```python
from build123d import *

# Parameters (mm, degrees)
F0_R     = 117.5
F1_DEPTH = 12.5
F3_DEPTH = 12.5
F4_COUNT = 4


with BuildPart() as f1:
    # F0 (on Front) → F1 (new body, symmetric)
    with BuildSketch(Plane.XZ):
        Circle(F0_R)
    extrude(amount=F1_DEPTH, both=True)

    # F2 (on Front) → F3 (cut, symmetric)
    with BuildSketch(Plane.XZ):
        with BuildLine():
            Line((7.3289173795, 97.9024141661), (11.9843448736, 116.8872340247))
            ThreePointArc((11.9843448736, 116.8872340247), (0, 117.5), (-11.9843448736, 116.8872340247))
            Line((-11.9843448736, 116.8872340247), (-7.3289173795, 97.9024141661))
            ThreePointArc((-7.3289173795, 97.9024141661), (-5.5587216743, 95.1591403196), (-2.4727905872, 94.0932258964))
            Line((-2.4727905872, 94.0932258964), (2.4727905872, 94.0932258964))
            ThreePointArc((2.4727905872, 94.0932258964), (5.5587216743, 95.1591403196), (7.3289173795, 97.9024141661))
        make_face()
    f3 = extrude(amount=F3_DEPTH, both=True, mode=Mode.SUBTRACT)

    # F4: F3 ×4 about axis
    f4_axis = Axis((0, 0, 0), (0, -1, 0))
    for i in range(1, F4_COUNT):
        add(f3.rotate(f4_axis, i * 360 / F4_COUNT), mode=Mode.SUBTRACT)


solid = f1.part
```
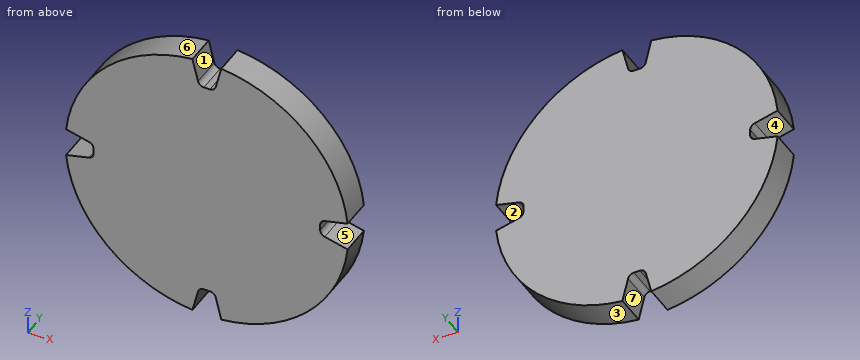
Can you work these out from the model? Positions are in its coordinate system, mm. Face numbers are marked on the shaded views. A direction names the side the tool comes from. Coordinates: 2 decimals unless noted, no trailing zeros. Loops run counter-clockwise (first coordinate to the right, second up) from the corner with the lowest first, then second, coordinate; pieces in that order, holes last.
1) For pin 1 (2.5 mm diameter, centred on y = -1, z = -0.5, fed in from -X); pin 2 (5 mm diameter, centred on x = 60.5, y = -9, fed in from +Z); pin 3 (2 mm diameter, centred on x = 74, y = 1.5, fed in from +Z), each with a flat end and sliding along its axis, tell me the tip position at first contact or that it passes through.
2) Thinking about a two-plate mould opening in X: for the marked faces 5, 6 and 7, which applies, pulls with the +X half, pulls with the -X half, needs draft (parallel to the pull), parting line crosses it, or undercut?
3) Imagine slicing it at C-C on z = 72. List the corners of the cut face in (x, y) for me, plus the area to 3 significant figures.
4) I need wall thicknesses on probe 1 along X at (y, z) = (-7.25, 1.5); probe 2 along Z at (x, y) = (107.5, 10.5); probe 3 along X at (y, z) = (-8.5, 106). Which ranges of each line are inside material? Lowest first, please.
5) Which directions (+Z, -Z, +X, -X, +Y, -Y) give clear straight access to the entire face, cutting with the end or side of a thin tool? Please do the marked faces 1, 2, 3 and 4.
6) Imagine slicing it at B-B on x = 39.5. List the corners of the cut face in (y, z) for me, plus the area to 3 significant figures.
7) Imagine slicing it at A-A on y = -9.25. List the corners of the cut face in (x, z) for me, plus the area to 3 significant figures.
Completed:
1. pin 1: stops at x = -94.09
1. pin 2: stops at z = 102.19
1. pin 3: stops at z = 92.07
2. face 5: pulls with the +X half
2. face 6: pulls with the -X half
2. face 7: undercut
3. outline: (-92.86, -12.5) - (92.86, -12.5) - (92.86, 12.5) - (-92.86, 12.5) - close
3. area: 4,640 mm2
4. probe 1: x = -94.09 to 94.09
4. probe 2: z = -47.43 to -9.68, 9.68 to 47.43
4. probe 3: x = -50.7 to -9.31, 9.31 to 50.7
5. face 1: +Z, +Y, -Y
5. face 2: +X, +Y, -Y
5. face 3: -Z, +X, +Y, -Y
5. face 4: -X, +Y, -Y
6. outline: (-12.5, -110.66) - (12.5, -110.66) - (12.5, 110.66) - (-12.5, 110.66) - close
6. area: 5,530 mm2
7. outline: (-116.89, -11.98) arc R117.5 ccw to (-11.98, -116.89) - (-7.33, -97.9) arc R5 cw to (-2.47, -94.09) - (2.47, -94.09) arc R5 cw to (7.33, -97.9) - (11.98, -116.89) arc R117.5 ccw to (116.89, -11.98) - (97.9, -7.33) arc R5 cw to (94.09, -2.47) - (94.09, 2.47) arc R5 cw to (97.9, 7.33) - (116.89, 11.98) arc R117.5 ccw to (11.98, 116.89) - (7.33, 97.9) arc R5 cw to (2.47, 94.09) - (-2.47, 94.09) arc R5 cw to (-7.33, 97.9) - (-11.98, 116.89) arc R117.5 ccw to (-116.89, 11.98) - (-97.9, 7.33) arc R5 cw to (-94.09, 2.47) - (-94.09, -2.47) arc R5 cw to (-97.9, -7.33) - close
7. area: 41,700 mm2
